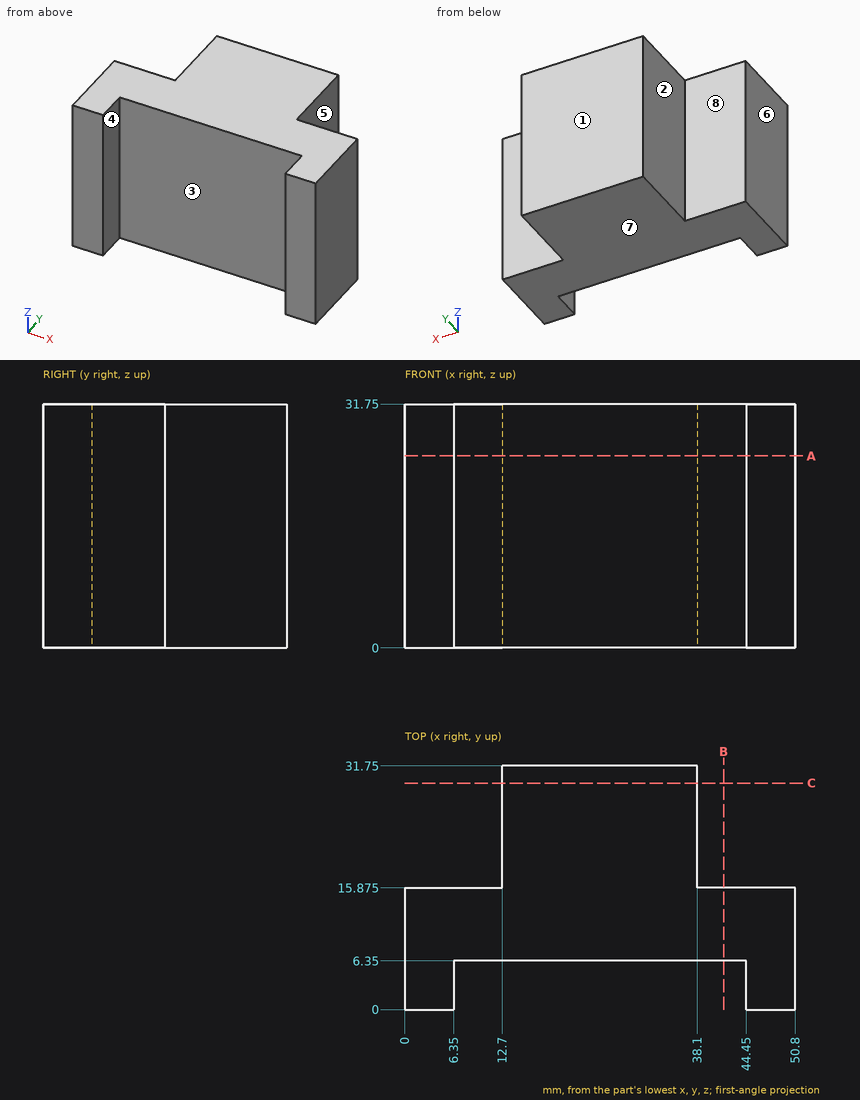
Could you check a few things on this drawing? It's one solid part, dimensions in mm from its lowest x, y, z. A direction names the side the tool comes from. Round coordinates to 2 decimals unless told otherwise and drop trailing zeros. Write each loop counter-clockwise with the first axis right and the second up, starting at its lowest first coordinate (ties: lowest second). Pieces come first, ordered by that corner, then holes. Notation, with made-up numbers: M 77,-36.75 L 108,-36.75 A23 cw 108,-13.75 Z; hole C -22.75,5 d11. An arc over 180 degrees is marked long. Answer as CSV lines item,"result". Start each with the question number.
1. Suppose I cut it at B-B on x = 41.5. Write out the boundary of the cut face in (y, z) (3 decimals).
2. Suppose I cut it at A-A on z = 25. Write out the boundary of the cut face in (x, y) (3 decimals), then the cut area to 3 significant figures.
3. On a 3-axis mill with a long thin cutter (end or side, diameter ignored), from which of +Z, -Z, +X, -X, +Y, -Y can I reach the whole of each face in a straight line? I mean the marked faces 4, 5, 6, 7 and 8. Say none if no direction works.
4. Suppose I cut it at C-C on y = 29.5. Write out the boundary of the cut face in (x, z).
5. I'm going to push flat-ended pins straight in: pin 1 Ø1.5 at (x, y) = (10.5, 22) entering from +Z; pin 2 Ø9.5 at (x, z) = (20, 11) entering from -Y; pin 3 Ø4 at (x, z) = (43.5, 18) entering from +Y (3 decimals). Where does each tip first touch, or does it pass through?
6. Thinking about a two-plate mould opening in X: for the marked faces 1, 2 and 3, which applies, released by +X, released by -X, zero draft, split by the parting line, or undercut?
7. I need wall thicknesses on probe 1 along X at (y, z) = (4.5, 14); probe 2 along Y at (x, z) = (17.5, 22.5); probe 3 along X at (y, z) = (21, 24.5). Which ranges of each line are inside material? Lowest first, please.
Check result:
1,outline,"M 6.35,0 L 15.875,0 L 15.875,31.75 L 6.35,31.75 Z"
2,outline,"M 0,0 L 6.35,0 L 6.35,6.35 L 44.45,6.35 L 44.45,0 L 50.8,0 L 50.8,15.875 L 38.1,15.875 L 38.1,31.75 L 12.7,31.75 L 12.7,15.875 L 0,15.875 Z"
2,area,"968 mm2"
3,face 4,"+Z, -Z, -Y"
3,face 5,"+Z, -Z, +X, +Y"
3,face 6,"+Z, -Z, -X, +Y, -Y"
3,face 7,"-Z, +X, -X, +Y, -Y"
3,face 8,"+Z, -Z, -X, +Y"
4,outline,"M 12.7,0 L 38.1,0 L 38.1,31.75 L 12.7,31.75 Z"
5,pin 1,"passes through"
5,pin 2,"stops at y = 6.35"
5,pin 3,"stops at y = 15.875"
6,face 1,"zero draft"
6,face 2,"released by -X"
6,face 3,"undercut"
7,probe 1,"x = 0 to 6.35, 44.45 to 50.8"
7,probe 2,"y = 6.35 to 31.75"
7,probe 3,"x = 12.7 to 38.1"
